```python
from build123d import *

# Parameters (mm, degrees)
BOSS_EXTRUDE2_DEPTH = 50.8


with BuildPart() as part:
    # Sketch3 → Boss-Extrude2 (new body)
    with BuildSketch(Plane.XY.offset(50.8)):
        Polygon((-1384.025, 292.740485768), (937.968055241, -398.75), (952.775, -398.75), (952.775, -297.15), (-1384.025, 398.75), align=None)
    extrude(amount=BOSS_EXTRUDE2_DEPTH)


solid = part.part
```
Can you work these out from the model? Positions are in its coordinate system, mm. Give positions to 0.01 mm unless a question says otherwise; leave off trailing zeros. Order: outer loops, then holes, each group sorted by start corner. A loop starts at its lowest first (then second) coordinate and runs counter-clockwise, first axis right, second up. Notation, with made-up numbers: (-27.5, 38.25) - (-20.5, 38.25) arc R3 cw to (-20.5, 42.25) - close; hole circle Ø4 at (35.25, 22). An arc over 180 degrees is marked (long way). Use a Markdown table: item, result. Add a question column.
Q1. If we section it at A-A on z = 59: Write out the boundary of the cut face in (x, y) (3 decimals), plus the area to 3 significant figures.
Q2. If we section it at B-B on x = -639.5: Write out the boundary of the cut face in (y, z).
Q3. I'm going to push a flat-ended pin straight in: pin 1 (1.5 mm diameter, centred on x = -491, z = 88.5, fed in from +Y). Where does the tip first touch, or does it pass through?
Q4. If we section it at C-C on y = 76.5: Write out the boundary of the cut face in (x, z).
Q5. If we mould it in two halves opening along Z, with no side actions, what happens to faces 1 (the flat face through (-199.27, 45.93, 75.84)), 2 (the flat face through (-221, 2, 50.8)), 3 (the flat face through (-221, 2, 101.6))? For each: released by +Z, released by -Z, zero draft, split by the parting line, or undercut.
Q6. Please list where these lines run through material, in increasing order: line 1 along Y through (x, z) = (56, 61); line 2 along Y through (x, z) = (37.5, 69).
Answers follow:
| question | item | result |
|---|---|---|
| 1 | outline | (-1384.025, 292.74) - (937.968, -398.75) - (952.775, -398.75) - (952.775, -297.15) - (-1384.025, 398.75) - close |
| 1 | area | 248,000 mm^2 |
| 2 | outline | (71.02, 50.8) - (177.03, 50.8) - (177.03, 101.6) - (71.02, 101.6) - close |
| 3 | pin 1 | stops at y = 133.03 |
| 4 | outline | (-657.9, 50.8) - (-301.92, 50.8) - (-301.92, 101.6) - (-657.9, 101.6) - close |
| 5 | face 1 | zero draft |
| 5 | face 2 | released by -Z |
| 5 | face 3 | released by +Z |
| 6 | line 1 | y = -136.1 to -30.09 |
| 6 | line 2 | y = -130.59 to -24.58 |
